For this review, take the finished solid that the model builds, in its own axes (mm). Face numbers are marked on the shaded views. A direction names the side the tool comes from. Give positions to 0.01 mm unless a question says otherwise; leave off trailing zeros. Loops run counter-clockwise (first coordinate to the right, second up) from the corner with the lowest first, then second, coordinate; pieces in that order, holes last.
```python
from build123d import *

# Parameters (mm, degrees)
BOSS_EXTRUDE1_DEPTH      = 4.44
BOSS_EXTRUDE1_DEPTH_BACK = 6
SKETCH21_W               = 19.5
SKETCH21_H               = 24
CUT_EXTRUDE2_DEPTH       = 24.71192527
CUT_EXTRUDE2_DEPTH_BACK  = 24.71192527
SKETCH14_R               = 1
CUT_EXTRUDE4_DEPTH       = 23.650882985
CUT_EXTRUDE4_DEPTH_BACK  = 23.650882985
SKETCH20_W               = 31.709739698
SKETCH20_H               = 13.674781638
SKETCH23_W               = 10
SKETCH23_H               = 3
CUT_EXTRUDE5_DEPTH       = 1.9
FILLET1_R                = 1.5
FILLET2_R                = 1.5


with BuildPart() as part:
    # Sketch21 → Boss-Extrude1 (new, two sides: drawn at the far end of the back side and taken through both)
    with BuildSketch(Plane(origin=(0, 0, 0), x_dir=(1, 0, 0), z_dir=(0, 1, 0)).offset(-BOSS_EXTRUDE1_DEPTH_BACK)):
        with Locations((8.5, 0)):
            Rectangle(SKETCH21_W, SKETCH21_H)
    extrude(amount=BOSS_EXTRUDE1_DEPTH + BOSS_EXTRUDE1_DEPTH_BACK)

    # Sketch14 → Cut-Extrude2 (cut, two sides: drawn at the far end of the back side and taken through both)
    with BuildSketch(Plane(origin=(0, 3.23, 0), x_dir=(1, 0, 0), z_dir=(0, 1, 0)).offset(-CUT_EXTRUDE2_DEPTH_BACK)):
        with Locations(Location((4.75, 0, 0), (0, 0, 270))):
            Circle(SKETCH14_R)
        with Locations(Location((7.25, 0, 0), (0, 0, 270))):
            Circle(SKETCH14_R)
        with Locations(Location((9.75, 0, 0), (0, 0, 270))):
            Circle(SKETCH14_R)
        with Locations(Location((12.25, 0, 0), (0, 0, 270))):
            Circle(SKETCH14_R)
    extrude(amount=CUT_EXTRUDE2_DEPTH + CUT_EXTRUDE2_DEPTH_BACK, mode=Mode.SUBTRACT)

    # Sketch20 → Cut-Extrude4 (cut, two sides: drawn at the far end of the back side and taken through both)
    with BuildSketch(Plane(origin=(0, 0, 0), x_dir=(0, 0, -1), z_dir=(1, 0, 0)).offset(-CUT_EXTRUDE4_DEPTH_BACK)):
        with Locations((-0.27698472, -0.290016026)):
            Rectangle(SKETCH20_W, SKETCH20_H)
        with BuildLine():
            Line((-4.4, -0.36), (-4.4, -3.26))
            Line((-4.4, -3.26), (-6.4, -3.26))
            Line((-6.4, -3.26), (-6.4, 4.14))
            Line((-6.4, 4.14), (9.7, 4.14))
            Line((9.7, 4.14), (9.7, -3.36))
            Line((9.7, -3.36), (5.7, -3.36))
            Line((5.7, -3.36), (5.7, -0.36))
            ThreePointArc((5.7, -0.36), (4.821320344, 1.761320344), (2.7, 2.64))
            Line((2.7, 2.64), (0, 2.64))
            Line((0, 2.64), (-1.4, 2.64))
            ThreePointArc((-1.4, 2.64), (-3.521320344, 1.761320344), (-4.4, -0.36))
        make_face(mode=Mode.SUBTRACT)
    extrude(amount=CUT_EXTRUDE4_DEPTH + CUT_EXTRUDE4_DEPTH_BACK, mode=Mode.SUBTRACT)

    # Sketch23 → Cut-Extrude5 (cut)
    with BuildSketch(Plane(origin=(0, 4.14, 0), x_dir=(1, 0, 0), z_dir=(0, 1, 0))):
        with Locations((8.5, 5.7)):
            Rectangle(SKETCH23_W, SKETCH23_H)
    extrude(amount=-CUT_EXTRUDE5_DEPTH, mode=Mode.SUBTRACT)

    # Fillet1
    fillet1_edges = [part.edges().sort_by_distance(p)[0] for p in [
        (8.5, 2.24, -7.2),
        (8.5, 2.24, -4.2),
    ]]
    fillet(fillet1_edges, radius=FILLET1_R - 0.0001)  # a hair under: the kernel refuses the full size

    # Fillet2
    fillet2_edges = [part.edges().sort_by_distance(p)[0] for p in [
        (3.5, 3.93995, -4.2),
        (3.5, 3.93995, -7.2),
        (3.5, 2.679310539, -6.760689461),
        (13.5, 3.93995, -7.2),
        (13.5, 3.93995, -4.2),
        (13.5, 2.679310539, -4.639310539),
        (3.5, 2.679310539, -4.639310539),
        (13.5, 2.679310539, -6.760689461),
    ]]
    fillet(fillet2_edges, radius=FILLET2_R - 0.0001)  # a hair under: the kernel refuses the full size


solid = part.part
```
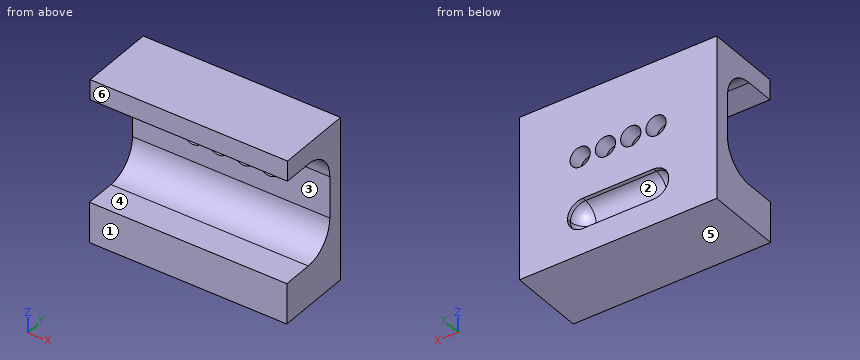
Item 1: For L1, parallel to X at y = 3.25, z = 0; L2, parallel to Z at x = 7.25, y = 3.75; L3, parallel to Z at x = 4, y = -2.5, list the stretches that pass through material, from the lowest coordinate up.
Answer:
L1: x = -1.25 to 3.75, 5.75 to 6.25, 8.25 to 8.75, 10.75 to 11.25, 13.25 to 18.25
L2: z = -9.7 to -7.2, -4.2 to -1, 1 to 6.4
L3: z = -9.7 to -5.7, 4.4 to 6.4
Item 2: The part is to be moulded in two halves that separate along Z. For the marked faces 4, 5 and 6, say which applies: released by +Z, released by -Z, zero draft, split by the parting line, or undercut.
Answer:
face 4: undercut
face 5: released by -Z
face 6: zero draft
Item 3: Take a section at C-C on z = 0. Give the boundary of the cut face in (x, y), and give its area (4 significant figures).
Answer:
outline: (-1.25, 2.64) - (3.75, 2.64) - (3.75, 4.14) - (-1.25, 4.14) - close; (5.75, 2.64) - (6.25, 2.64) - (6.25, 4.14) - (5.75, 4.14) - close; (8.25, 2.64) - (8.75, 2.64) - (8.75, 4.14) - (8.25, 4.14) - close; (10.75, 2.64) - (11.25, 2.64) - (11.25, 4.14) - (10.75, 4.14) - close; (13.25, 2.64) - (18.25, 2.64) - (18.25, 4.14) - (13.25, 4.14) - close
area: 17.25 mm2
Item 4: Take a section at B-B on y = -2. Give the boundary of the cut face in (x, z).
Answer:
outline: (-1.25, -9.7) - (18.25, -9.7) - (18.25, -5.7) - (-1.25, -5.7) - close; (-1.25, 4.4) - (18.25, 4.4) - (18.25, 6.4) - (-1.25, 6.4) - close
Item 5: Clearance check with flat-ended pins moving along their axes: pin 1 Ø2.5 at (x, z) = (4.75, 0) entering from -Y; pin 2 Ø6 at (x, z) = (11.5, 0.5) entering from +Y; pin 3 Ø1.8 at (x, z) = (9.75, 0) entering from -Y; pin 4 Ø1 at (x, z) = (9.5, 5) entering from -Y. State where each tip first meets the part, or that it passes through.
Answer:
pin 1: stops at y = 2.64
pin 2: stops at y = 4.14
pin 3: passes through
pin 4: stops at y = -3.26
Item 6: Take a section at D-D on x = 1.25. Give the boundary of the cut face in (y, z).
Answer:
outline: (-3.36, -9.7) - (4.14, -9.7) - (4.14, 6.4) - (-3.26, 6.4) - (-3.26, 4.4) - (-0.36, 4.4) arc R3 cw to (2.64, 1.4) - (2.64, -2.7) arc R3 cw to (-0.36, -5.7) - (-3.36, -5.7) - close
Item 7: Tool access review of the marked faces 1, 2 and 3: name each direction out of +Z, -Z, +X, -X, +Y, -Y from which nothing blocks a thin tool from reaching the whole face with its end or side.
Answer:
face 1: +Z, -Z, +X, -X, -Y
face 2: +Y
face 3: +X, -X, -Y
